Model file for the job. Use its own axes, mm. A direction names the side the tool comes from. Coordinates: 2 decimals unless noted, no trailing zeros. One line per question, with ' | ' between items. Start each with the question number.
(1) Wall check: probe 1 along Z at (x, y) = (2, -26); probe 2 along X at (y, z) = (-25.5, -16); probe 3 along Z at (x, y) = (-2, -3). Give the ranges that are in metal, low to high.
(2) Flat gauge pins, fed straight in: pin 1 Ø10 at (x, y) = (76.5, -17) entering from -Z; pin 2 Ø2.5 at (x, z) = (-63.5, -64.5) entering from +Y; pin 3 Ø1.5 at (x, y) = (31, -21.5) entering from -Z; pin 4 Ø10 at (x, z) = (62, 62.5) entering from +Y. Where does each tip first touch, or does it go through?
(3) Two-plate mould, pull along Y, no slides. Class faces 1 (the face through (-62, -0.938, -44)), 2 (the face through (-23.19, 1.49, -30.24)), 3 (the face through (64, 2.012, 64)): +Y half, -Y half, draft (parallel to the pull), parting line (faces both ways), or undercut.
(4) Tool access for faces 4 (the face through (31, -2.938, -71)), 5 (the face through (47, -30.938, -47)), 6 (the face through (3.33, -27.99, -10.56)): list every direction of +Z, -Z, +X, -X, +Y, -Y with a clear straight run to the whole face (end or side of a thin tool).
from build123d import *

# Parameters (mm, degrees)
SKETCH2_R                 = 50
BOSS_EXTRUDE1_DEPTH       = 10
SKETCH8_R                 = 17.55
CUT_EXTRUDE4_DEPTH        = 5.05
SKETCH12_R                = 3.25
CUT_EXTRUDE7_DEPTH        = 71.890778667
SKETCH13_R                = 5.5
CUT_EXTRUDE8_DEPTH        = 2
SKETCH14_R                = 15
SKETCH14_R_2              = 3.25
BOSS_EXTRUDE3_DEPTH       = 7.5
CHAMFER1_SIZE             = 7.5
SKETCH15_R                = 5.1
CUT_EXTRUDE9_DEPTH        = 2.5
CHAFL_N2_SIZE             = 0.5
SKETCH16_R                = 25
SKETCH16_R_2              = 22
CUT_EXTRUDE10_DEPTH       = 3.2
CHAMFER2_SIZE             = 0.1
CHAMFER3_SIZE             = 0.25
CHAMFER5_SIZE             = 0.25
SCALE1_SCALE              = 2.1714285
BOSS_EXTRUDE4_START       = -17.3714281
BOSS_EXTRUDE4_OUTLINE_R   = 108.571425
BOSS_EXTRUDE4_OUTLINE_R_2 = 57.926200599
BOSS_EXTRUDE4_DEPTH       = 17.3714281
BOSS_EXTRUDE5_START       = -5
SKETCH17_3_R              = 100.830783289
SKETCH17_3_R_2            = 57.926200599
BOSS_EXTRUDE5_DEPTH       = 5
CUT_EXTRUDE11_DEPTH       = 5.05
CIRPATTERN1_COUNT         = 4
CUT_EXTRUDE12_START       = -13
CUT_EXTRUDE12_DEPTH       = 29
BOSS_EXTRUDE6_START       = -8
BOSS_EXTRUDE6_DEPTH       = 8
CUT_EXTRUDE13_DEPTH       = 20
BOSS_EXTRUDE7_START       = 2
BOSS_EXTRUDE7_DEPTH       = 2
CIRPATTERN2_COUNT         = 4
CIRPATTERN3_COUNT         = 4


# Read off the part's stored shape, not the designer's step: Boss-Extrude4
with BuildPart() as part:
    # Sketch2 → Boss-Extrude1 (new body)
    with BuildSketch(Plane(origin=(0, 0, 0), x_dir=(1, 0, 0), z_dir=(0, 1, 0))):
        with Locations(Location((0, 0, 0), (0, 0, 270))):
            Circle(SKETCH2_R)
    extrude(amount=-BOSS_EXTRUDE1_DEPTH)

    # Sketch8 → Cut-Extrude4 (cut)
    with BuildSketch(Plane(origin=(0, 0, 0), x_dir=(1, 0, 0), z_dir=(0, 1, 0))):
        with Locations(Location((0, 0, 0), (0, 0, 270))):
            Circle(SKETCH8_R)
    extrude(amount=-CUT_EXTRUDE4_DEPTH, mode=Mode.SUBTRACT)

    # Sketch12 → Cut-Extrude7 (cut, through all)
    with BuildSketch(Plane(origin=(0, -5.05, 0), x_dir=(1, 0, 0), z_dir=(0, 1, 0))):
        with Locations(Location((0, 0, 0), (0, 0, 270))):
            Circle(SKETCH12_R)
    extrude(amount=-CUT_EXTRUDE7_DEPTH, mode=Mode.SUBTRACT)

    # Sketch13 → Cut-Extrude8 (cut)
    with BuildSketch(Plane(origin=(0, -5.05, 0), x_dir=(1, 0, 0), z_dir=(0, 1, 0))):
        with Locations(Location((0, 0, 0), (0, 0, 270))):
            Circle(SKETCH13_R)
    extrude(amount=-CUT_EXTRUDE8_DEPTH, mode=Mode.SUBTRACT)

    # Sketch14 → Boss-Extrude3 (add)
    with BuildSketch(Plane.XZ.offset(10)):
        with Locations(Location((0, 0, 0), (0, 0, 90))):
            Circle(SKETCH14_R)
        with Locations(Location((0, 0, 0), (0, 0, 90))):
            Circle(SKETCH14_R_2, mode=Mode.SUBTRACT)
    extrude(amount=BOSS_EXTRUDE3_DEPTH)

    # Chamfer1
    chamfer1_edges = [part.edges().sort_by_distance(p)[0] for p in [
        (0, -10, -15),
    ]]
    chamfer(chamfer1_edges, length=CHAMFER1_SIZE - 0.0001)  # a hair under: the kernel refuses the full size

    # Sketch15 → Cut-Extrude9 (cut)
    with BuildSketch(Plane.XZ.offset(17.5)):
        with Locations(Location((0, 0, 0), (0, 0, 270))):
            Circle(SKETCH15_R)
    extrude(amount=-CUT_EXTRUDE9_DEPTH, mode=Mode.SUBTRACT)

    # Chaflán2
    chafl_n2_edges = [part.edges().sort_by_distance(p)[0] for p in [
        (0, 0, -50),
        (0, -10, -50),
    ]]
    chamfer(chafl_n2_edges, length=CHAFL_N2_SIZE)

    # Sketch16 → Cut-Extrude10 (cut)
    with BuildSketch(Plane(origin=(0, 0, 0), x_dir=(1, 0, 0), z_dir=(0, 1, 0))):
        with Locations(Location((0, 0, 0), (0, 0, 270))):
            Circle(SKETCH16_R)
        with Locations(Location((0, 0, 0), (0, 0, 270))):
            Circle(SKETCH16_R_2, mode=Mode.SUBTRACT)
    extrude(amount=-CUT_EXTRUDE10_DEPTH, mode=Mode.SUBTRACT)

    # Chamfer2
    chamfer2_edges = [part.edges().sort_by_distance(p)[0] for p in [
        (0, -3.2, -25),
        (0, -3.2, -22),
        (0, -5.05, -17.55),
    ]]
    chamfer(chamfer2_edges, length=CHAMFER2_SIZE)

    # Chamfer3
    chamfer3_edges = [part.edges().sort_by_distance(p)[0] for p in [
        (0, -5.05, -5.5),
        (0, -7.05, -3.25),
        (0, 0, -25),
        (0, 0, -22),
        (0, 0, -17.55),
    ]]
    chamfer(chamfer3_edges, length=CHAMFER3_SIZE)

    # Chamfer5
    chamfer5_edges = [part.edges().sort_by_distance(p)[0] for p in [
        (0, -17.5, 5.1),
        (0, -15, -3.25),
    ]]
    chamfer(chamfer5_edges, length=CHAMFER5_SIZE)


with BuildPart() as part_1:
    # Scale1: scaled about (0, -6.02867632, 0)
    add(part.part.scale(SCALE1_SCALE).moved(Location((0, 7.062163259, 0))))

    # Boss-Extrude4 outline → Boss-Extrude4 (add)
    with BuildSketch(Plane.XZ.offset(30.93782581).offset(BOSS_EXTRUDE4_START)):
        Circle(BOSS_EXTRUDE4_OUTLINE_R)
        Circle(BOSS_EXTRUDE4_OUTLINE_R_2, mode=Mode.SUBTRACT)
    extrude(amount=BOSS_EXTRUDE4_DEPTH)

    # Sketch17<3> → Boss-Extrude5 (add)
    with BuildSketch(Plane.XZ.offset(30.93782581).offset(BOSS_EXTRUDE5_START)):
        Circle(SKETCH17_3_R)
        with Locations(Location((0, 0, 0), (0, 0, 270))):
            Circle(SKETCH17_3_R_2, mode=Mode.SUBTRACT)
    extrude(amount=BOSS_EXTRUDE5_DEPTH)

    # Sketch18 → Cut-Extrude11 (cut)
    with BuildSketch(Plane(origin=(0, 7.06217294, 0), x_dir=(1, 0, 0), z_dir=(0, 1, 0))):
        Polygon((-65.009306884, 68.356942866), (-68.356942866, 65.009306884), (-67.131623054, 60.43635109), (-62.55866726, 59.211031278), (-59.211031278, 62.55866726), (-60.43635109, 67.131623054), align=None)
    cut_extrude11 = extrude(amount=-CUT_EXTRUDE11_DEPTH, mode=Mode.SUBTRACT)

    # CirPattern1: Cut-Extrude11 ×4 about axis
    cirpattern1_axis = Axis((0, 0, 0), (0, 1, 0))
    for i in range(1, CIRPATTERN1_COUNT):
        add(cut_extrude11.rotate(cirpattern1_axis, i * 360 / CIRPATTERN1_COUNT), mode=Mode.SUBTRACT)

    # Sketch19 → Cut-Extrude12 (cut)
    with BuildSketch(Plane(origin=(0, 0, 0), x_dir=(1, 0, 0), z_dir=(0, 1, 0)).offset(CUT_EXTRUDE12_START)):
        with BuildLine():
            Line((-79.4, 0), (-60.6, 0))
            ThreePointArc((-60.6, 0), (-55.98709967, 23.190616001), (-42.85067094, 42.85067094))
            Line((-42.85067094, 42.85067094), (-43.15860775, 43.15860775))
            Line((-43.15860775, 43.15860775), (-56.144278426, 56.144278426))
            ThreePointArc((-56.144278426, 56.144278426), (-73.356034881, 30.38506453), (-79.4, 0))
        make_face()
    cut_extrude12 = extrude(amount=CUT_EXTRUDE12_DEPTH, mode=Mode.SUBTRACT)

    # Sketch20 → Boss-Extrude6 (add)
    with BuildSketch(Plane(origin=(0, 7.06217294, 0), x_dir=(1, 0, 0), z_dir=(0, 1, 0)).offset(BOSS_EXTRUDE6_START)):
        with BuildLine():
            Line((-56.187341587, 22.701159561), (-73.618398053, 29.743763517))
            ThreePointArc((-73.618398053, 29.743763517), (-66.210534272, 43.823796634), (-56.144278426, 56.144278426))
            Line((-56.144278426, 56.144278426), (-42.85067094, 42.85067094))
            ThreePointArc((-42.85067094, 42.85067094), (-50.533480817, 33.44738131), (-56.187341587, 22.701159561))
        make_face()
    boss_extrude6 = extrude(amount=BOSS_EXTRUDE6_DEPTH)

    # Sketch21 → Cut-Extrude13 (cut)
    with BuildSketch(Plane(origin=(0, 7.06217294, 0), x_dir=(1, 0, 0), z_dir=(0, 1, 0))):
        with BuildLine():
            Line((-45.961940777, 45.961940777), (-53.033008589, 53.033008589))
            ThreePointArc((-53.033008589, 53.033008589), (-62.541436655, 41.395273898), (-69.538789093, 28.095494506))
            Line((-69.538789093, 28.095494506), (-60.266950547, 24.349428572))
            ThreePointArc((-60.266950547, 24.349428572), (-54.202578434, 35.875904045), (-45.961940777, 45.961940777))
        make_face()
    cut_extrude13 = extrude(amount=-CUT_EXTRUDE13_DEPTH, mode=Mode.SUBTRACT)

    # Sketch22 → Boss-Extrude7 (add)
    with BuildSketch(Plane.XZ.offset(0.93782706).offset(BOSS_EXTRUDE7_START)):
        with BuildLine():
            Line((-58.561646908, -28.205203623), (-54.597473887, -26.295928301))
            ThreePointArc((-54.597473887, -26.295928301), (-55.421561016, -24.511437627), (-56.187341587, -22.701159561))
            Line((-56.187341587, -22.701159561), (-60.266950547, -24.349428572))
            ThreePointArc((-60.266950547, -24.349428572), (-59.445568746, -26.29114597), (-58.561646908, -28.205203623))
        make_face()
        with BuildLine():
            ThreePointArc((-67.571131048, -32.544465719), (-68.591040861, -30.335937658), (-69.538789093, -28.095494506))
            Line((-69.538789093, -28.095494506), (-73.618398053, -29.743763517))
            ThreePointArc((-73.618398053, -29.743763517), (-72.615048592, -32.115646), (-71.535304069, -34.453741041))
            Line((-71.535304069, -34.453741041), (-67.571131048, -32.544465719))
        make_face()
    boss_extrude7 = extrude(amount=-BOSS_EXTRUDE7_DEPTH)

    # CirPattern2: Cut-Extrude12, Boss-Extrude6, Cut-Extrude13 ×4 about axis
    cirpattern2_axis = Axis((0, 6.519315815, 0), (0, 1, 0))
    add([cut_extrude12.rotate(cirpattern2_axis, i * 360 / CIRPATTERN2_COUNT) for i in range(1, CIRPATTERN2_COUNT)], mode=Mode.SUBTRACT)
    add([boss_extrude6.rotate(cirpattern2_axis, i * 360 / CIRPATTERN2_COUNT) for i in range(1, CIRPATTERN2_COUNT)])
    add([cut_extrude13.rotate(cirpattern2_axis, i * 360 / CIRPATTERN2_COUNT) for i in range(1, CIRPATTERN2_COUNT)], mode=Mode.SUBTRACT)

    # CirPattern3: Boss-Extrude7 ×4 about axis
    cirpattern3_axis = Axis((0, -8.246397985, 0), (0, 1, 0))
    for i in range(1, CIRPATTERN3_COUNT):
        add(boss_extrude7.rotate(cirpattern3_axis, i * 360 / CIRPATTERN3_COUNT))


solid = part_1.part
Filled in:
1) probe 1: -108.55 to -57.89, -37.46 to -10.89, 10.89 to 37.46, 57.89 to 108.55 | probe 2: -107.39 to -55.67, -34.48 to 34.48, 55.67 to 107.39 | probe 3: -108.55 to -38.06, 38.06 to 60.57, 79.37 to 108.55
2) pin 1: z = -81.7 | pin 2: y = 2.01 | pin 3: z = -104.27 | pin 4: y = 7.06
3) face 1: undercut | face 2: draft | face 3: +Y half
4) face 4: none | face 5: +Z, -Z, +X, -X, -Y | face 6: -Y
